```python
from build123d import *

# Parameters (mm, degrees)
SKETCH1_R               = 4.5
SKETCH1_R_2             = 3
BOSS_EXTRUDE1_DEPTH     = 6
SKETCH2_R               = 1.5
CUT_EXTRUDE1_DEPTH      = 1
CUT_EXTRUDE1_DEPTH_BACK = 21


with BuildPart() as part:
    # Sketch1 → Boss-Extrude1 (new body)
    with BuildSketch(Plane.XY):
        with BuildLine():
            Line((-10, 0), (0, 0))
            Line((0, 0), (10, 0))
            Line((10, 0), (10, 14.38749457))
            ThreePointArc((10, 14.38749457), (4.456626225, 12.796504363), (8.312500108, 17.085149749))
            ThreePointArc((8.312500108, 17.085149749), (2.5e-08, 19), (-8.312500062, 17.085149771))
            ThreePointArc((-8.312500062, 17.085149771), (-5.409009772, 16.930868332), (-4, 14.38749457))
            ThreePointArc((-4, 14.38749457), (-7, 11.38749457), (-10, 14.38749457))
            Line((-10, 14.38749457), (-10, 0))
        make_face()
        with Locations((0, 11)):
            Circle(SKETCH1_R, mode=Mode.SUBTRACT)
        with Locations((7, 14.38749457)):
            Circle(SKETCH1_R_2)
        with Locations((-7, 14.38749457)):
            Circle(SKETCH1_R_2)
        with BuildLine():
            Line((10, 0), (0, 0))
            Line((0, 0), (-10, 0))
            Line((-10, 0), (-10, -14.38749457))
            ThreePointArc((-10, -14.38749457), (-7, -11.38749457), (-4, -14.38749457))
            ThreePointArc((-4, -14.38749457), (-5.409009694, -16.930868283), (-8.312499897, -17.085149852))
            ThreePointArc((-8.312499897, -17.085149852), (9.1e-08, -19), (8.312500061, -17.085149772))
            ThreePointArc((8.312500061, -17.085149772), (4.456626238, -12.796504341), (10, -14.38749457))
            Line((10, -14.38749457), (10, 0))
        make_face()
        with Locations((0, -11)):
            Circle(SKETCH1_R, mode=Mode.SUBTRACT)
        with Locations((-7, -14.38749457)):
            Circle(SKETCH1_R_2)
        with Locations((7, -14.38749457)):
            Circle(SKETCH1_R_2)
    extrude(amount=BOSS_EXTRUDE1_DEPTH)

    # Sketch2 → Cut-Extrude1 (cut, two sides)
    with BuildSketch(Plane(origin=(10, 0, 0), x_dir=(0, 0, -1), z_dir=(1, 0, 0))) as cut_extrude1_sk:
        with Locations((-3, 11)):
            Circle(SKETCH2_R)
        with Locations((-3, -11)):
            Circle(SKETCH2_R)
    extrude(amount=CUT_EXTRUDE1_DEPTH, mode=Mode.SUBTRACT)
    extrude(cut_extrude1_sk.sketch, amount=-CUT_EXTRUDE1_DEPTH_BACK, mode=Mode.SUBTRACT)


solid = part.part
```
Input: part model. Units: mm. Frame: model coordinates. Coordinates: 2 decimals unless noted, no trailing zeros. Order: outer loops, then holes, each group sorted by start corner. A loop starts at its lowest first (then second) coordinate and runs counter-clockwise, first axis right, second up. Notation, with made-up numbers: (72, 19) - (99, 19) arc R21 cw to (99, 32) - close; hole circle Ø1 at (56, -1). An arc over 180 degrees is marked (long way). Put each result on its own line as item: value.
1. Draft query along Y for faces 1 (the face through (9.53, -16, 2.96)), 2 (the face through (0, 0, 0)), 3 (the face through (-7.081, 10.425, 1.614)). Return one class per face: pulls with the +Y half, pulls with the -Y half, needs draft (parallel to the pull), parting line crosses it, or undercut.
Report:
face 1: pulls with the -Y half
face 2: needs draft
face 3: undercut
2. Line query: line 1 along Y through (x, z) = (-0.25, 2.5); line 2 along Z through (x, y) = (-6.7, -11); line 3 along Y through (x, z) = (1, 3.75). Output: solid intervals per line, ascending.
Report:
line 1: y = -19 to -15.49, -6.51 to 6.51, 15.49 to 19
line 2: z = 0 to 1.5, 4.5 to 6
line 3: y = -18.97 to -15.39, -6.61 to 6.61, 15.39 to 18.97
3. Cut plane C-C on x = 0.5. Return the cut outline in (y, z).
Report:
outline: (-18.99, 0) - (-15.47, 0) - (-15.47, 6) - (-18.99, 6) - close; (-6.53, 0) - (6.53, 0) - (6.53, 6) - (-6.53, 6) - close; (15.47, 0) - (18.99, 0) - (18.99, 6) - (15.47, 6) - close
4. Cut plane D-D on z = 3.75. Return the cut outline in (x, y).
Report:
outline: (-10, -14.39) arc R3 ccw to (-8.31, -17.09) arc R19 ccw to (8.31, -17.09) arc R3 ccw to (10, -14.39) - (10, -12.3) - (4.31, -12.3) arc R4.5 cw to (-4.31, -12.3) - (-10, -12.3) - close; (-10, -9.7) - (-4.31, -9.7) arc R4.5 cw to (4.31, -9.7) - (10, -9.7) - (10, 9.7) - (4.31, 9.7) arc R4.5 cw to (-4.31, 9.7) - (-10, 9.7) - close; (-10, 12.3) - (-4.31, 12.3) arc R4.5 cw to (4.31, 12.3) - (10, 12.3) - (10, 14.39) arc R3 ccw to (8.31, 17.09) arc R19 ccw to (-8.31, 17.09) arc R3 ccw to (-10, 14.39) - close
5. Contact query for flat-ended pins moving along their axis: pin 1 Ø12 at (x, y) = (1.5, -10.5) entering from -Z; pin 2 Ø2.5 at (y, z) = (11, 3) entering from -X. Output: stop coordinate, or through.
Report:
pin 1: stops at z = 0
pin 2: passes through
6. Cut plane A-A on z = 1. Return the cut outline in (x, y).
Report:
outline: (-10, -14.39) arc R3 ccw to (-8.31, -17.09) arc R19 ccw to (8.31, -17.09) arc R3 ccw to (10, -14.39) - (10, 14.39) arc R3 ccw to (8.31, 17.09) arc R19 ccw to (-8.31, 17.09) arc R3 ccw to (-10, 14.39) - close; hole circle Ø9 at (0, -11); hole circle Ø9 at (0, 11)
7. Cut plane B-B on y = -11. Return the cut outline in (x, z), then the cut area to 3 significant figures.
Report:
outline: (-10, 0) - (-4.5, 0) - (-4.5, 1.5) - (-10, 1.5) - close; (-10, 4.5) - (-4.5, 4.5) - (-4.5, 6) - (-10, 6) - close; (4.5, 0) - (10, 0) - (10, 1.5) - (4.5, 1.5) - close; (4.5, 4.5) - (10, 4.5) - (10, 6) - (4.5, 6) - close
area: 33.0 mm2
